Geometry: final body of the model. Coordinates: model frame, mm. Face numbers are marked on the shaded views. A direction names the side the tool comes from. Give positions to 0.01 mm unless a question says otherwise; leave off trailing zeros. Order: outer loops, then holes, each group sorted by start corner. A loop starts at its lowest first (then second) coordinate and runs counter-clockwise, first axis right, second up. Notation, with made-up numbers: (-24.5, 14.5) -> (15.5, 14.5) arc R28 ccw to (15.5, 42.5) -> close; hole circle Ø4 at (-5.75, 28). An arc over 180 degrees is marked (long way). Answer in a Markdown table with one row per item. Add a question column.
Q1. Cut plane B-B on x = 15. Return the cut outline in (y, z), and give its area (3 significant figures).
Q2. Cut plane C-C on z = 13.5. Return the cut outline in (x, y), and give its area (3 significant figures).
Q3. Line query: line 1 along Z through (x, y) = (-13, 10.5); line 2 along Z through (x, y) = (0, -13); line 3 along Z through (x, y) = (5, -4.5). Output: solid intervals per line, ascending. Write a range as from..to.
Q4. Cut plane A-A on y = 16. Return the cut outline in (x, z).
Q5. Pull-direction query (X, two-part tool) for the marked faces 4, 5 and 6; classes: +X half, -X half, draft (parallel to the pull), parting line (faces both ways), or undercut.
Q6. Set-up query: the marked faces 1, 2 and 3. Return all of +Z, -Z, +X, -X, +Y, -Y with unobstructed straight access to the full face (end or side cutting, diameter ignored); none if empty.
Q7. Cut plane D-D on x = 7.5. Return the cut outline in (y, z).
Q8. Contact query for flat-ended pins moving along their axis: P1, Ø1, axis at x = -3.5, z = 13.5, coming from the +Y side; P2, Ø3, axis at x = -9.5, z = 2, coming from the -Y side; P3, Ø18.5, axis at x = 1.5, y = -3, coming from the -Z side; P4, Ø3, axis at y = -15, z = 18.5, coming from the -X side. Output: stop coordinate, or through.
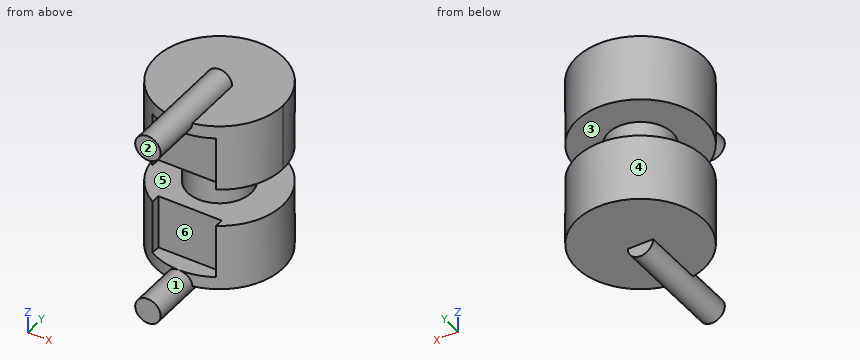
from build123d import *

# Parameters (mm, degrees)
F0_R          = 20
F1_DEPTH      = 27
F2_W          = 19.3877541561
F2_H          = 12
F5_R          = 4
F6_DEPTH      = 35.2
F7_W          = 20
F7_H          = 11.4580463721
F8_DEPTH      = 17
F8_DEPTH_BACK = 29


with BuildPart() as f1:
    # F0 (on Top) → F1 (new body, symmetric)
    with BuildSketch(Plane.XY):
        Circle(F0_R)
    extrude(amount=F1_DEPTH, both=True)

    # F2 (on Front) → F4 (revolve, cut)
    with BuildSketch(Plane.XZ):
        with Locations((19.6938770781, 0)):
            Rectangle(F2_W, F2_H)
    revolve(axis=Axis((0, 0, 0.1814514399), (0, 0, -1)), mode=Mode.SUBTRACT)

    # F5 (on Front) → F6 (join)
    with BuildSketch(Plane.XZ):
        with Locations((0, 27)):
            Circle(F5_R)
        with Locations((0, -27)):
            Circle(F5_R)
    extrude(amount=F6_DEPTH)

    # F7 (on face) → F8 (cut, two sides)
    with BuildSketch(Plane.XY.offset(-6)) as f8_sk:
        with Locations((0, -20.229023186)):
            Rectangle(F7_W, F7_H)
    extrude(amount=-F8_DEPTH, mode=Mode.SUBTRACT)
    extrude(f8_sk.sketch, amount=F8_DEPTH_BACK, mode=Mode.SUBTRACT)


solid = f1.part
Completed:
| question | item | result |
|---|---|---|
| 1 | outline | (-13.23, -27) -> (13.23, -27) -> (13.23, -6) -> (-13.23, -6) -> close; (-13.23, 6) -> (13.23, 6) -> (13.23, 27) -> (-13.23, 27) -> close |
| 1 | area | 1,110 mm² |
| 2 | outline | (-10, -17.32) -> (-10, -14.5) -> (10, -14.5) -> (10, -17.32) arc R20 ccw (long way) to start |
| 2 | area | 1,160 mm² |
| 3 | line 1 | z = -27..-6, 6..27 |
| 3 | line 2 | z = -31..-6, 6..31 |
| 3 | line 3 | z = -27..27 |
| 4 | outline | (-12, -27) -> (12, -27) -> (12, -6) -> (-12, -6) -> close; (-12, 6) -> (12, 6) -> (12, 27) -> (-12, 27) -> close |
| 5 | face 4 | parting line |
| 5 | face 5 | draft |
| 5 | face 6 | undercut |
| 6 | face 1 | -Y |
| 6 | face 2 | +Z, -Z, +X, -X, -Y |
| 6 | face 3 | none |
| 7 | outline | (-18.54, -27) -> (18.54, -27) -> (18.54, -6) -> (6.61, -6) -> (6.61, 6) -> (18.54, 6) -> (18.54, 27) -> (-18.54, 27) -> (-18.54, 23) -> (-14.5, 23) -> (-14.5, 6) -> (-6.61, 6) -> (-6.61, -6) -> (-14.5, -6) -> (-14.5, -23) -> (-18.54, -23) -> close |
| 8 | P1 | stops at y = 19.77 |
| 8 | P2 | stops at y = -6 |
| 8 | P3 | stops at z = -31 |
| 8 | P4 | stops at x = -14.76 |
